from build123d import *

# Parameters (mm, degrees)
F0_W        = 49.9999988824
F0_H        = 29.9999988824
F0_W_2      = 45.8000008941
F0_H_2      = 25.8000008941
F0_W_3      = 45.0000008941
F0_H_3      = 25.0000008941
F0_W_4      = 40
F0_H_4      = 20
F1_DEPTH    = 30
F2_DEPTH    = 25
F3_T1_DEPTH = 45


# Not quite as in the source:
# - a fillet or chamfer that OpenCascade refuses, or shapes differently, is made with other operations: its cross-section is extruded or revolved along the edge and cut away or added


with BuildPart() as f1:
    # F0 (on Top) → F1 (new body)
    with BuildSketch(Plane.XY):
        Rectangle(F0_W, F0_H)
        Rectangle(F0_W_2, F0_H_2, mode=Mode.SUBTRACT)
        Rectangle(F0_W_2, F0_H_2)
        Rectangle(F0_W_3, F0_H_3, mode=Mode.SUBTRACT)
        Rectangle(F0_W_3, F0_H_3)
        Rectangle(F0_W_4, F0_H_4, mode=Mode.SUBTRACT)
        Rectangle(F0_W_4, F0_H_4)
    extrude(amount=F1_DEPTH)

    # F0 (on Top) → F2 (cut)
    with BuildSketch(Plane.XY):
        Rectangle(F0_W_2, F0_H_2)
        Rectangle(F0_W_3, F0_H_3, mode=Mode.SUBTRACT)
        Rectangle(F0_W_3, F0_H_3)
        Rectangle(F0_W_4, F0_H_4, mode=Mode.SUBTRACT)
        Rectangle(F0_W_4, F0_H_4)
    extrude(amount=F2_DEPTH, mode=Mode.SUBTRACT)

    # F3: fillet of radius 3 on 4 edges, made by hand

    # F3_s2 → F3_t1 (cut)
    with BuildSketch(Plane.XY.offset(-7.5)):
        with BuildLine():
            add(Edge.make_bspline(
                [(-21.9999994412, -14.9999994412), (-24.9999994412, -14.9999994412), (-24.9999994412, -11.9999994412)],
                knots=[0, 0, 0, 1, 1, 1], degree=2, weights=[1, 1, 1]))
            Line((-24.9999994412, -11.9999994412), (-24.9999994412, -14.9999994412))
            Line((-24.9999994412, -14.9999994412), (-21.9999994412, -14.9999994412))
        make_face()
        with BuildLine():
            add(Edge.make_bspline(
                [(-24.9999994412, 11.9999994412), (-24.9999994412, 14.9999994412), (-21.9999994412, 14.9999994412)],
                knots=[0, 0, 0, 1, 1, 1], degree=2, weights=[1, 1, 1]))
            Line((-21.9999994412, 14.9999994412), (-24.9999994412, 14.9999994412))
            Line((-24.9999994412, 14.9999994412), (-24.9999994412, 11.9999994412))
        make_face()
        with BuildLine():
            add(Edge.make_bspline(
                [(21.9999994412, -14.9999994412), (24.9999994412, -14.9999994412), (24.9999994412, -11.9999994412)],
                knots=[0, 0, 0, 1, 1, 1], degree=2, weights=[1, 1, 1]))
            Line((24.9999994412, -11.9999994412), (24.9999994412, -14.9999994412))
            Line((24.9999994412, -14.9999994412), (21.9999994412, -14.9999994412))
        make_face()
        with BuildLine():
            add(Edge.make_bspline(
                [(24.9999994412, 11.9999994412), (24.9999994412, 14.9999994412), (21.9999994412, 14.9999994412)],
                knots=[0, 0, 0, 1, 1, 1], degree=2, weights=[1, 1, 1]))
            Line((21.9999994412, 14.9999994412), (24.9999994412, 14.9999994412))
            Line((24.9999994412, 14.9999994412), (24.9999994412, 11.9999994412))
        make_face()
    extrude(amount=F3_T1_DEPTH, mode=Mode.SUBTRACT)


solid = f1.part
Read the model definition and answer for the solid it produces. Units are mm, in the model's axes. A direction names the side the tool comes from. Round coordinates to 2 decimals unless told otherwise and drop trailing zeros. Write each loop counter-clockwise with the first axis right and the second up, starting at its lowest first coordinate (ties: lowest second). Pieces come first, ordered by that corner, then holes. Notation, with made-up numbers: (18, 69.5) - (37, 69.5) arc R28 ccw to (37, 91.5) - close; hole circle Ø3 at (6, 59.25). An arc over 180 degrees is marked (long way). Use a Markdown table: item, result.
(1) The mould has two halves that part along X. Classify faces 1 (the flat face through (-25, 0, 15)), 2 (the flat face through (0, -12.9, 12)), 3 (the flat face through (25, 0, 15)): released by +X, released by -X, zero draft, split by the parting line, or undercut.
Reported:
| item | result |
|---|---|
| face 1 | released by -X |
| face 2 | undercut |
| face 3 | released by +X |
(2) The part is cut by section B-B (y = 9.25). Write down the section's boundary in (x, z), then the cut area to 3 significant figures.
Reported:
| item | result |
|---|---|
| outline | (-25, 0) - (-22.9, 0) - (-22.9, 25) - (22.9, 25) - (22.9, 0) - (25, 0) - (25, 30) - (-25, 30) - close |
| area | 355 mm2 |
(3) The part is cut by section A-A (x = 4.5). Write down the section's boundary in (y, z).
Reported:
| item | result |
|---|---|
| outline | (-15, 0) - (-12.9, 0) - (-12.9, 25) - (12.9, 25) - (12.9, 0) - (15, 0) - (15, 30) - (-15, 30) - close |
(4) Which of the six approach directions +Z, -Z, +X, -X, +Y, -Y give full straight-line access (tool end or side, diameter ignored) to faces 4 (the flat face through (-0.1, -13.3, 0)), 5 (the flat face through (-22.9, 0, 12))?
Reported:
| item | result |
|---|---|
| face 4 | -Z, +X, -X, +Y, -Y |
| face 5 | -Z |
(5) Straight lines are drawn through the part: line 1 along X through (y, z) = (5.75, 3.5); line 2 along Y through (x, z) = (-12, 22.5); line 3 along Z through (x, y) = (-0.5, 12.25). For each, find the intervals that lie inside material, in ascending order. Write a range as [from, to].
Reported:
| item | result |
|---|---|
| line 1 | [-25, -22.9], [22.9, 25] |
| line 2 | [-15, -12.9], [12.9, 15] |
| line 3 | [25, 30] |
